Autodesk Inventor part; units mm, degrees
ref_plane "YZ Plane" through (0, 0, 0) normal (1, 0, 0) x (0, 1, 0)
ref_plane "XZ Plane" through (0, 0, 0) normal (0, 1, 0) x (-1, 0, 0)
ref_plane "XY Plane" through (0, 0, 0) normal (0, 0, 1) x (1, 0, 0)
sketch "Sketch1" plane through (0, 0, 0) normal (0, 0, 1) x (1, 0, 0)
  line L0 (0, 571.5) -> (0, -571.5) construction
  line L1 (-6.5, 571.5) -> (-6.5, -571.5)
  line L2 (6.5, -571.5) -> (6.5, 571.5)
  arc A0 (6.5, 571.5) -> (-6.5, 571.5) centre (0, 571.5) ccw
  arc A1 (-6.5, -571.5) -> (6.5, -571.5) centre (0, -571.5) ccw
  line L3 (-4.5, 571.5) -> (-4.5, -571.5)
  arc A2 (-4.5, -571.5) -> (4.5, -571.5) centre (0, -571.5) ccw
  line L4 (4.5, -571.5) -> (4.5, 571.5)
  arc A3 (4.5, 571.5) -> (-4.5, 571.5) centre (0, 571.5) ccw
  line L5 (-8.5, 571.5) -> (-8.5, -571.5)
  arc A4 (-8.5, -571.5) -> (8.5, -571.5) centre (0, -571.5) ccw
  line L6 (8.5, -571.5) -> (8.5, 571.5)
  arc A5 (8.5, 571.5) -> (-8.5, 571.5) centre (0, 571.5) ccw
  point P0 (0, 0)
  dimension "d0" = 9
  dimension "d2" = 2
  dimension "d3" = 2
  dimension "d4" = 1143
extrude "Extrusion1" add sketch "Sketch1" along normal mid plane 4 contours A0 L2 A1 L1 | A5 L6 A4 L5
fillet "Fillet1" radius 2 16 edges at (0, -580, 2) (8.5, 0, 2) (0, 580, 2) (-8.5, 0, 2) (0, 576, 2) (4.5, 0, 2) (0, -576, 2) (-4.5, 0, 2) (0, -576, -2) (4.5, 0, -2) (0, 576, -2) (-4.5, 0, -2) (0, 580, -2) (8.5, 0, -2) (0, -580, -2) (-8.5, 0, -2)
properties part number "REVLIFT-Test String" material "Nylon 6"
Verification items for the finished model (mm, model axes). Round coordinates to 2 decimals unless told otherwise and drop trailing zeros. Write each loop counter-clockwise with the first axis right and the second up, starting at its lowest first coordinate (ties: lowest second). Pieces come first, ordered by that corner, then holes.
1. Section check C-C on z = 0.75. Enter the section's corners in (x, y), plus the area to 3 significant figures.
2. Scan lines: L1, parallel to X at y = 368, z = -0.75; L2, parallel to X at y = -275, z = -0.85; L3, parallel to Y at x = -0.5, z = -0.5. Record each from-to range of solid material in increasing order.
3. Gauge pin test, flat ends, axial feed: P1, Ø5, axis at x = -3, y = 437, coming from the +Z side; P2, Ø4, axis at x = -4, y = -116.5, coming from the -Z side. Record the tip position at first contact, or that the pin passes through.
Answer:
1. outline: (-8.35, -571.5) arc R8.35 ccw to (8.35, -571.5) - (8.35, 571.5) arc R8.35 ccw to (-8.35, 571.5) - close; hole (-4.65, -571.5) arc R4.65 ccw to (4.65, -571.5) - (4.65, 571.5) arc R4.65 ccw to (-4.65, 571.5) - close
1. area: 8,630 mm2
2. L1: x = -8.35 to -4.65, 4.65 to 8.35
2. L2: x = -8.31 to -4.69, 4.69 to 8.31
2. L3: y = -579.92 to -576.04, 576.04 to 579.92
3. P1: stops at z = 1.73
3. P2: stops at z = -1.94
